Source: CAD feature listing. Evaluate the final solid. Frame: model axes, mm. Face numbers are marked on the shaded views. A direction names the side the tool comes from. Coordinates: 2 decimals unless noted, no trailing zeros. Loops run counter-clockwise (first coordinate to the right, second up) from the corner with the lowest first, then second, coordinate; pieces in that order, holes last.
Item 1: Section query A-A, the plane y = 36. Return the cut outline in (x, z).
Item 2: Section query D-D, the plane y = 9. Return the cut outline in (x, z).
Item 3: Section query C-C, the plane z = 35.5. State how many separate pieces and enclosed holes the cut face has, then the cut area to 3 significant figures.
Item 4: Pin query (flat end, axial travel): pin 1 Ø1.5 at (y, z) = (12.5, 9.5) entering from +X; pin 2 Ø8 at (x, z) = (109.5, 28) entering from -Y; pin 3 Ø8 at (y, z) = (25.5, 4.5) entering from -X. Return the tip coordinate at first contact, or that it passes through.
Item 5: Reachability of the marked faces 1, 2 and 3 from +Z, -Z, +X, -X, +Y, -Y: full face, straight path, thin tool, end or side. Return the list, or none.
Item 6: Section query B-B, the plane y = -25.15. Return the cut outline in (x, z), then the cut area to 3 significant figures.
Item 7: Pull-direction query (Y, two-part tool) for the marked faces 4, 5 and 6; classes: +Y half, -Y half, draft (parallel to the pull), parting line (faces both ways), or undercut.
Item 8: Line query: probe 1 along Y at (x, z) = (142.5, 32.5); probe 2 along Y at (x, z) = (129, 32.5); probe 3 along X at (y, z) = (38.5, 6.9). Output: solid intervals per line, ascending.
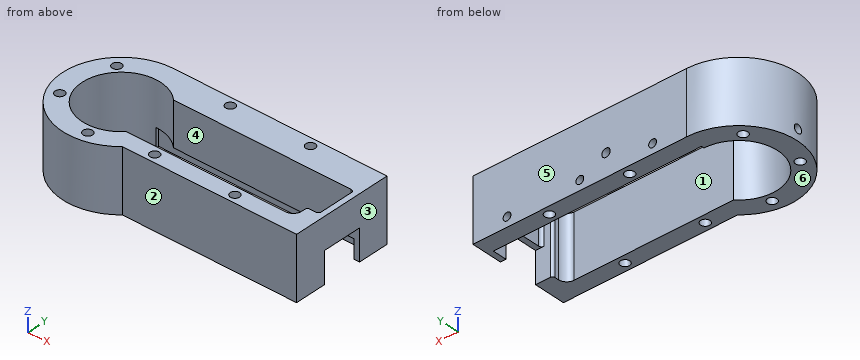
Autodesk Inventor part; units mm, degrees
ref_plane "Work Plane1" through (0, 0, 12) normal (0, 0, -1) x (-1, 0, 0)
ref_plane "Work Plane2" through (-23.5188, -31.15, 0) normal (1, 0, 0) x (0, 0, -1)
ref_plane "Work Plane3" through (0, 0, 22.274) normal (0, 0, -1) x (-1, 0, 0)
sketch "Sketch1" plane through (0, 0, 0) normal (0, 0, 1) x (1, 0, 0)
  circle A0 centre (0, 0) radius 11.1125 construction
  line L0 (104.364, -18.65) -> (70.364, -18.65) construction
  line L1 (104.364, 18.65) -> (70.364, 18.65) construction
  line L2 (23.9529, -7.067) -> (23.9529, 14.933) construction
  arc A1 (-39, 0) -> (23.4665, -31.15) centre (0, 0) ccw construction
  line L3 (50.614, 19.35) -> (60.114, 19.35) construction
  line L4 (50.614, 19.85) -> (60.114, 19.85)
  line L5 (60.114, -18.65) -> (50.614, -18.65) construction
  arc A2 (19.7478, 19.85) -> (20.4274, -19.15) centre (0, 0) ccw
  line L6 (0, 42) -> (171.45, 42)
  line L7 (-238.861, -48) -> (171.45, -48) construction
  line L8 (-39, 0) -> (-42, 0) construction
  arc A3 (0, 42) -> (28.1723, -31.15) centre (0, 0) ccw
  circle A4 centre (0, 0) radius 14.224
  line L9 (171.45, 42) -> (171.45, -31.15)
  line L10 (19.7478, 19.85) -> (152.6937, 19.85)
  line L11 (152.6937, -19.15) -> (20.4274, -19.15)
  line L12 (23.4665, -31.15) -> (171.45, -31.15)
  line L13 (0, 28) -> (0, 30)
  line L14 (0, 30) -> (117.475, 30)
  line L15 (142.2077, -8.6311) -> (152.6937, -8.6311)
  line L16 (117.475, 30) -> (117.475, 19.85) construction
  line L17 (117.475, -19.15) -> (117.475, -31.15)
  line L18 (140.3854, -10.4534) -> (140.3854, -13.15)
  line L19 (148.6937, 19.85) -> (148.6937, -6.6311)
  line L20 (117.475, 30) -> (171.45, 30) construction
  line L21 (-34.4683, 6.0777) -> (0, 0) construction
  line L22 (-22.4976, -26.8116) -> (0, 0) construction
  line L23 (0, 0) -> (11.9707, -32.8892) construction
  circle A5 centre (0, 0) radius 34 construction
  line L24 (117.475, 19.85) -> (148.6937, 19.85)
  line L25 (148.6937, 19.85) -> (148.6937, 30)
  line L26 (152.6937, 30) -> (117.475, 30)
  line L27 (117.475, 30) -> (117.475, 19.85) construction
  line L28 (34.114, 20.2591) -> (34.114, 32) construction
  line L29 (65.364, 20.2591) -> (65.364, 32) construction
  line L30 (33.864, 19.85) -> (33.864, 32) construction
  line L31 (65.614, 19.85) -> (65.614, 32) construction
  line L32 (22.4976, 36) -> (171.45, 36) construction
  line L33 (171.45, -25.15) -> (28.0371, -25.15) construction
  circle A6 centre (-24.2686, 23.8125) radius 3.35
  circle A7 centre (-30.1464, -15.7223) radius 3.35
  circle A8 centre (5.6371, -33.5294) radius 3.35
  circle A9 centre (33.6303, -5) radius 3.35
  circle A10 centre (15.1476, 30.4393) radius 3.35
  circle A11 centre (46.0375, 36) radius 3.35
  circle A12 centre (46.0375, -25.15) radius 3.35
  circle A13 centre (136.0375, 36) radius 3.35
  circle A14 centre (136.0375, -25.15) radius 3.35
  arc A15 (146.6937, -8.6311) -> (148.6937, -6.6311) centre (146.6937, -6.6311) ccw
  arc A16 (142.2077, -8.6311) -> (140.3854, -10.4534) centre (142.2077, -10.4534) ccw
  arc A17 (148.6937, 28) -> (146.6937, 30) centre (146.6937, 28) ccw
  line L34 (152.6937, 42) -> (152.6937, -31.15)
  line L35 (148.6937, 11.5374) -> (171.45, 11.5374)
  line L36 (171.45, 11.5374) -> (171.45, -8.6311)
  line L37 (171.45, -8.6311) -> (152.6937, -8.6311)
  line L38 (148.6937, -8.6435) -> (148.6937, 11.5374)
  circle A18 centre (103.364, 36) radius 3.35
  circle A19 centre (103.364, -25.15) radius 3.35
  line L39 (140.3854, -10.4534) -> (140.3854, -0.553)
  line L40 (142.3854, 1.447) -> (148.6937, 1.447)
  arc A20 (142.3854, 1.447) -> (140.3854, -0.553) centre (142.3854, -0.553) ccw
  arc A21 (134.3854, -19.15) -> (140.3854, -13.15) centre (134.3854, -13.15) ccw
  line L41 (140.747, -6.35) -> (140.747, 7.9375) construction
  arc A22 (148.6937, 17.85) -> (146.6937, 19.85) centre (146.6937, 17.85) ccw
  arc A23 (146.6937, 19.85) -> (148.6937, 21.85) centre (146.6937, 21.85) ccw
  point P0 (171.45, -22)
  point P1 (140.3854, -8.6311)
  point P2 (171.45, -7.65)
  point P3 (171.45, 7)
  point P4 (148.6937, -8.6311)
  point P5 (33.864, 30)
  point P6 (65.614, 30)
  point P7 (140.2077, 19.85)
  point P8 (148.6937, 17.7587)
  point P9 (152.6937, 11.5374)
  point P10 (152.6937, -8.6435)
  point P11 (148.6937, -8.6311)
  dimension "d38" = 68
  dimension "d0" = 78
  dimension "d4" = 0.5
  dimension "d6" = 56
  dimension "d8" = 90
  dimension "d9" = 28.448
  dimension "d12" = 12
  dimension "d23" = 12
  dimension "d24" = 0.5
  dimension "d25" = 38
  dimension "d27" = 42
  dimension "d33" = 80
  dimension "d36" = 39
  dimension "d37" = 28
  dimension "d39" = 6
  dimension "d49" = 0.25
  dimension "d50" = 0.25
  dimension "d55" = 6
  dimension "d56" = 6.7
  dimension "d59" = 360
  dimension "d62" = 6.7
  dimension "d65" = 90
  dimension "d70" = 171.45
  dimension "d84" = 2
  dimension "d92" = 4
  dimension "d102" = 2
  dimension "d111" = 6
  dimension "d116" = 4
  dimension "d117" = 2
extrude "Extrusion1" add sketch "Sketch1" along normal blind 28.448 contours A2 L11 L17 L12 A3 L6 L34 L26 L14 A10 L13 | L25 L26 L34 L10 | L11 L34 L12 L17 | A10 L14 | A21 L18 A16 L15 L34 L11 | A13 | A14 picked at (15.3429, 31.3449)
extrude "Extrusion2" add sketch "Sketch1" along normal blind 16.1 from surface at 28.448 contours L10 A2 L13 L14 A10 L26 A17 L25 A23 L4 | A2 L11 L17 L12 A3 L6 L34 L26 L14 A10 L13 | A23 L25 L10 | L25 L26 L34 L10 | L11 L34 L12 L17 | A10 L14 | L14 A10 | A17 L26 L25 | A21 L18 A16 L15 L34 L11 | A13 | A14
sketch "Sketch2" plane through (0, 42, 0) normal (0, 1, 0) x (1, 0, 0)
  circle A0 centre (24.3468, -37.648) radius 2.8
  line L0 (171.45, -43.548) -> (0, -43.548) construction
  line L1 (152.6937, 0) -> (0, 0)
  line L2 (0, 0) -> (0, -44.548)
  line L3 (0, -44.548) -> (152.6937, -44.548)
  line L4 (152.6937, 0) -> (152.6937, -44.548)
  circle A1 centre (76.3468, -37.648) radius 2.8
  circle A2 centre (128.3468, -37.648) radius 2.8
  line L5 (152.6937, 0) -> (152.6937, -44.548) construction
  line L6 (152.6937, -22.274) -> (0, -22.274) construction
  line L7 (0, 0) -> (0, -28.448) construction
  circle A3 centre (24.3468, -6.9) radius 2.8
  circle A4 centre (76.3468, -6.9) radius 2.8
  circle A5 centre (128.3468, -6.9) radius 2.8
  circle A6 centre (57.6393, -16.071) radius 3
  dimension "d73" = 5.6
  dimension "d93" = 24.3468
  dimension "d94" = 152.6937
  dimension "d97" = 52
  dimension "d108" = 6.9
extrude "Extrusion4" cut sketch "Sketch2" against normal blind 15.1 contours A3 | A4 | A5 | A6
ref_plane "Work Plane1" through (0, 0, 12) normal (0, 0, -1) x (-1, 0, 0)
sketch "Sketch6" plane through (152.6937, -31.15, 0) normal (1, 0, 0) x (0, 0, -1)
  line L0 (0, 30.597) -> (-28.448, 30.597)
  circle A0 centre (-7.9375, 30.597) radius 3
  dimension "d104" = 6
ref_plane "Work Plane2" through (-23.5188, -31.15, 0) normal (1, 0, 0) x (0, 0, -1)
extrude "Extrusion6" cut sketch "Sketch6" against normal blind 30 from surface at -176.2125
extrude "Extrusion7" add sketch "Sketch1" against normal blind 15.1 from surface at 28.448 contours L10 A2 L13 L14 A10 L26 A17 L25 A23 L4 | A23 L25 L10 | L14 A10 | A17 L26 L25 picked at (15.3464, 28.8029)
ref_plane "Work Plane3" through (0, 0, 22.274) normal (0, 0, -1) x (-1, 0, 0)
extrude "Extrusion8" add sketch "Sketch1" along normal up to surface (22.274 mm away) from surface at 22.274 contours L10 L19 A22 | L25 L26 L34 L10 | L10 L34 L35 L19 | L35 L34 L15 L38 L19 | A17 L26 L25 | L38 L15 A15
equation "\"d12\" = d23"
equation "\"d10\" = d9"
properties part number "Mech Panel v7 infill_01"
Verdict:
1. outline: (-21.63, 0) - (42.69, 0) - (42.69, 44.55) - (-21.63, 44.55) - close; (49.39, 0) - (100.01, 0) - (100.01, 44.55) - (49.39, 44.55) - close; (106.71, 0) - (152.69, 0) - (152.69, 44.55) - (106.71, 44.55) - close; hole circle Ø5.6 at (24.35, 6.9); hole circle Ø6 at (57.64, 16.07); hole circle Ø5.6 at (76.35, 6.9); hole circle Ø5.6 at (128.35, 6.9)
2. outline: (-41.02, 0) - (-26.51, 0) - (-26.51, 44.55) - (-41.02, 44.55) - close; (148.69, 22.27) - (152.69, 22.27) - (152.69, 44.55) - (148.69, 44.55) - close
3. separate pieces: 1
3. enclosed holes: 8
3. area: 6,730 mm2
4. pin 1: stops at x = -24.67
4. pin 2: stops at y = -31.15
4. pin 3: stops at x = -36.08
5. face 1: +Z, -Z
5. face 2: +Z, -Z, +X, -Y
5. face 3: +Z, -Z, +X, +Y, -Y
6. outline: (-33.64, 0) - (-12.31, 0) - (-12.31, 44.55) - (-33.64, 44.55) - close; (12.31, 0) - (42.69, 0) - (42.69, 44.55) - (12.31, 44.55) - close; (49.39, 0) - (100.01, 0) - (100.01, 44.55) - (49.39, 44.55) - close; (106.71, 0) - (152.69, 0) - (152.69, 44.55) - (106.71, 44.55) - close
6. area: 6,610 mm2
7. face 4: undercut
7. face 5: +Y half
7. face 6: draft
8. probe 1: y = -31.15 to -8.63, 19.85 to 42
8. probe 2: y = -31.15 to -19.15, 19.85 to 42
8. probe 3: x = -16.79 to 21.55, 27.15 to 43.81, 48.27 to 73.55, 79.15 to 101.13, 105.59 to 125.55, 131.15 to 152.69
